Solid Edge part; units mm, degrees
sketch "Sketch1" plane through (0, 0, 0) normal (1, 0, 0) x (0, 1, 0)
  line L0 (-15, 0) -> (-15, -4)
  line L1 (-15, -4) -> (-12.5, -4)
  line L2 (-12.5, -4) -> (-12.5, -2.5)
  line L3 (-12.5, -2.5) -> (12.5, -2.5)
  line L4 (12.5, -2.5) -> (12.5, -4)
  line L5 (12.5, -4) -> (15, -4)
  line L6 (15, -4) -> (15, 0)
  line L7 (15, 0) -> (-15, 0)
  dimension "D1" = 12.5
  dimension "D2" = 15
  dimension "D3" = 15
  dimension "D4" = 12.5
extrude "Protrusion1" add sketch "Sketch1" along normal mid plane 68
hole "Hole_1" at (0, -10, 0) direction (0, 0, -1) diameter 3.6 end up to next countersink diameter 6.94 countersink angle 90
hole "Hole1" at (0, 10, 0) direction (0, 0, -1) diameter 3.6 end up to next countersink diameter 6.94 countersink angle 90
chamfer "Chamfer_1" distance 10 angle 45 4 edges at (34, 15, -2) (34, -15, -2) (-34, 15, -2) (-34, -15, -2)
sketch "Sketch2" plane through (0, 0, 0) normal (0, 0, 1) x (1, 0, 0)
  line L0 (-7.5, -5) -> (7.5, -5)
  line L1 (7.5, -5) -> (7.5, 5)
  line L2 (7.5, 5) -> (-7.5, 5)
  line L3 (-7.5, 5) -> (-7.5, -5)
  dimension "D1" = 7.5
  dimension "D2" = 7.5
extrude "Cutout1" cut sketch "Sketch2" against normal up to next
sketch "Sketch3" plane through (0, 0, 0) normal (0, 0, 1) x (1, 0, 0)
  line L0 (-20.5, 0) -> (-14.7265, 10)
  line L1 (-14.7265, 10) -> (-11.7265, 10)
  line L2 (-11.7265, 10) -> (-17.5, 0)
  line L3 (-17.5, 0) -> (-11.7265, -10)
  line L4 (-11.7265, -10) -> (-14.7265, -10)
  line L5 (-14.7265, -10) -> (-20.5, 0)
  dimension "D1" = 14.7265
  dimension "D2" = 20.5
extrude "deco_cutout" cut sketch "Sketch3" against normal blind 0.5
pattern_linear "Pattern2" count 3 spacing 5 along (-1, 0, 0) of "deco_cutout"
mirror "Mirror1" about plane through (0, 0, 0) normal (1, 0, 0) of "deco_cutout", "Pattern2"
properties material "Polyethylene, low density"
Input: part model. Units: mm. Frame: model coordinates. A direction names the side the tool comes from. Coordinates: 2 decimals unless noted, no trailing zeros. Loops run counter-clockwise (first coordinate to the right, second up) from the corner with the lowest first, then second, coordinate; pieces in that order, holes last. Notation, with made-up numbers: (72, 36) - (80, 36) arc R16 ccw to (80, 55) - close; hole circle Ø2 at (36.25, 41.5). An arc over 180 degrees is marked (long way). Answer in a Markdown table with one row per item. Add a question column.
Item 1: Access query for faces 4 (the flat face through (0, -12.5, -3)), 5 (the flat face through (-22.4, -0.7, -0.5)), 6 (the flat face through (0, -5, -1)). Directions: +Z, -Z, +X, -X, +Y, -Y. A direction counts if a zero-diameter tool reaches every point of the face in a straight line with its end or side. Return the directions, or none.
Item 2: Contact query for flat-ended pins moving along their axis: P1, Ø1.5, axis at y = 9, z = -1, coming from the -X side; P2, Ø1, axis at y = -11, z = -0.5, coming from the +X side. Output: stop coordinate, or through.
Item 3: Section query C-C on x = 28.5. Return the cut outline in (y, z), then the cut area to 3 significant figures.
Item 4: Line query: line 1 along Y through (x, z) = (0, -2.05); line 2 along Y through (x, z) = (23, -3.7); line 3 along Y through (x, z) = (-17, -0.3). Output: solid intervals per line, ascending. Write a range as [from, to].
Item 5: Section query A-A on x = 0. Return the cut outline in (y, z).
Item 6: Mould query, pull axis X, two halves, no side actions, for faces 1 (the flat face through (-8, 0, 0)), 2 (the flat face through (-34, 0, -1)), 3 (the flat face through (22, 2, -0.5)). Classes: released by +X, released by -X, zero draft, split by the parting line, or undercut.
Recorded:
| question | item | result |
|---|---|---|
| 1 | face 4 | -Z, +X, -X |
| 1 | face 5 | +Z |
| 1 | face 6 | +Z, -Z |
| 2 | P1 | x = -30.75 |
| 2 | P2 | x = 28.5 |
| 3 | outline | (-10.5, -2.5) - (10.5, -2.5) - (10.5, 0) - (3.46, 0) - (3.46, -0.5) - (-3.46, -0.5) - (-3.46, 0) - (-10.5, 0) - close |
| 3 | area | 49.0 mm^2 |
| 4 | line 1 | [-15, -11.8], [-8.2, -5], [5, 8.2], [11.8, 15] |
| 4 | line 2 | [-15, -12.5], [12.5, 15] |
| 4 | line 3 | [-15, -10], [-9.53, -6.06], [-0.87, 0.87], [6.06, 9.53], [10, 15] |
| 5 | outline | (-15, -4) - (-12.5, -4) - (-12.5, -2.5) - (-11.8, -2.5) - (-11.8, -1.67) - (-13.47, 0) - (-15, 0) - close; (-8.2, -2.5) - (-5, -2.5) - (-5, 0) - (-6.53, 0) - (-8.2, -1.67) - close; (5, -2.5) - (8.2, -2.5) - (8.2, -1.67) - (6.53, 0) - (5, 0) - close; (11.8, -2.5) - (12.5, -2.5) - (12.5, -4) - (15, -4) - (15, 0) - (13.47, 0) - (11.8, -1.67) - close |
| 6 | face 1 | zero draft |
| 6 | face 2 | released by -X |
| 6 | face 3 | undercut |
